from build123d import *

# Parameters (mm, degrees)
F1_DEPTH = 15
F2_R     = 2.3
F3_R     = 2


with BuildPart() as f1:
    # F0 (on Top) → F1 (new body)
    with BuildSketch(Plane.XY):
        Polygon((-1.45, 8.5), (1.45, 8.5), (1.45, -8.5), (8, -8.5), (8, 16.5), (0, 16.5), (-8, 16.5), (-8, -8.5), (-1.45, -8.5), align=None)
    extrude(amount=F1_DEPTH)

    # F2
    f2_edges = [f1.edges().sort_by_distance(p)[0] for p in [
        (-1.45, 0, 15),
        (0, 8.5, 15),
        (1.45, 0, 15),
        (1.45, 0, 0),
        (0, 8.5, 0),
        (-1.45, 0, 0),
    ]]
    fillet(f2_edges, radius=F2_R)

    # F3
    f3_edges = [f1.edges().sort_by_distance(p)[0] for p in [
        (-5.875, -8.5, 15),
        (5.875, -8.5, 15),
    ]]
    fillet(f3_edges, radius=F3_R)


solid = f1.part
The listing builds one solid part. Answer for the finished solid, in the listing's coordinates (mm). A direction names the side the tool comes from. Give positions to 0.01 mm unless a question says otherwise; leave off trailing zeros. Loops run counter-clockwise (first coordinate to the right, second up) from the corner with the lowest first, then second, coordinate; pieces in that order, holes last. Notation, with made-up numbers: (11.25, -20) - (51.25, -20) arc R3 ccw to (51.25, -16) - close; hole circle Ø6 at (62.5, -26). An arc over 180 degrees is marked (long way). Use one line per item in the form item = value.
1. The mould has two halves that part along X. Classify faces 1 (the face through (5.9, -7.9, 14.43)), 2 (the face through (2.02, -7.9, 7.57)): pulls with the +X half, pulls with the -X half, needs draft (parallel to the pull), parting line crosses it, or undercut.
Calculated:
face_1 = needs draft
face_2 = undercut
2. Find the intervals of material crossed by line 1 along X through (y, z) = (-5.5, 8.5); line 2 along Y through (x, z) = (0.25, 11); line 3 along X through (y, z) = (-3, 2), in increasing order. Write a range as [from, to].
Calculated:
line_1 = [-8, -1.45], [1.45, 8]
line_2 = [8.5, 16.5]
line_3 = [-8, -1.47], [1.47, 8]
3. Which of the six approach directions +Z, -Z, +X, -X, +Y, -Y give full straight-line access (tool end or side, diameter ignored) to faces 3 (the face through (-2.1, 2.3, 0.7)), 4 (the face through (-2.05, -7.93, 7.43)), 5 (the face through (0.05, 9.46, 14.57))?
Calculated:
face_3 = -Z, -Y
face_4 = +Z, -Z, -Y
face_5 = +Z, -Y
4. Given pin 1 Ø6 at (x, z) = (2.5, 3.5) entering from -Y; pin 2 Ø2.5 at (x, z) = (0, 9.5) entering from -Y; pin 3 Ø2 at (x, y) = (1.5, 7) entering from -Z, each flat-ended and moving along its own axis, determine where each tip first touches the part or whether it passes through.
Calculated:
pin_1 = -8.5
pin_2 = 8.5
pin_3 = 0.37
5. Section C-C on x = 0.75 is taken. Give the vertices of the cut face in (y, z).
Calculated:
outline = (8.5, 2.3) arc R2.3 ccw to (10.8, 0) - (16.5, 0) - (16.5, 15) - (10.8, 15) arc R2.3 ccw to (8.5, 12.7) - close
6. Section B-B on z = 3.25 is taken. Give the vertices of the cut face in (x, y), then the cut area to 3 significant figures.
Calculated:
outline = (-8, -8.5) - (-3.45, -8.5) arc R2 ccw to (-1.45, -6.5) - (-1.45, 8.5) - (1.45, 8.5) - (1.45, -6.5) arc R2 ccw to (3.45, -8.5) - (8, -8.5) - (8, 16.5) - (-8, 16.5) - close
area = 349 mm^2
7. Section A-A on y = 2.5 is taken. Give the vertices of the cut face in (x, z), then the cut area to 3 significant figures.
Calculated:
outline = (-8, 0) - (-3.75, 0) arc R2.3 ccw to (-1.45, 2.3) - (-1.45, 12.7) arc R2.3 ccw to (-3.75, 15) - (-8, 15) - close; (1.45, 2.3) arc R2.3 ccw to (3.75, 0) - (8, 0) - (8, 15) - (3.75, 15) arc R2.3 ccw to (1.45, 12.7) - close
area = 192 mm^2
